Read the model definition and answer for the solid it produces. Units are mm, in the model's axes. A direction names the side the tool comes from. Give positions to 0.01 mm unless a question says otherwise; leave off trailing zeros. Order: outer loops, then holes, each group sorted by start corner. A loop starts at its lowest first (then second) coordinate and runs counter-clockwise, first axis right, second up.
```python
from build123d import *

# Parameters (mm, degrees)
F1_DEPTH = 63.5
F2_DEPTH = 25.4
F3_DEPTH = 8.255
F5_R     = 6.35


with BuildPart() as f1:
    # F0 (on Front) → F1 (new body, symmetric)
    with BuildSketch(Plane.XZ):
        Polygon((41.275, -9.525), (41.275, 9.525), (22.225, 9.525), (-41.275, 9.525), (-41.275, -9.525), align=None)
    extrude(amount=F1_DEPTH, both=True)

    # F0 (on Front) → F2 (join, symmetric)
    with BuildSketch(Plane.XZ):
        with BuildLine():
            Line((22.225, 9.525), (41.275, 9.525))
            Line((41.275, 9.525), (41.275, 27.0002))
            ThreePointArc((41.275, 27.0002), (45.166907, 37.412746), (54.934352, 42.719822))
            Line((54.934352, 42.719822), (54.934352, 61.854849))
            ThreePointArc((54.934352, 61.854849), (31.682991, 50.89972), (22.225, 27.0002))
            Line((22.225, 27.0002), (22.225, 9.525))
        make_face()
        with BuildLine():
            Line((54.934352, 61.854849), (54.934352, 42.719822))
            ThreePointArc((54.934352, 42.719822), (56.039455, 42.836308), (57.15, 42.8752))
            Line((57.15, 42.8752), (85.725, 42.8752))
            Line((85.725, 42.8752), (85.725, 61.9252))
            Line((85.725, 61.9252), (57.15, 61.9252))
            ThreePointArc((57.15, 61.9252), (56.041618, 61.907608), (54.934352, 61.854849))
        make_face()
    extrude(amount=F2_DEPTH, both=True)

    # F0 (on Front) → F3 (join, symmetric)
    with BuildSketch(Plane.XZ):
        with BuildLine():
            Line((-41.275, 9.525), (22.225, 9.525))
            Line((22.225, 9.525), (22.225, 27.0002))
            ThreePointArc((22.225, 27.0002), (31.682991, 50.89972), (54.934352, 61.854849))
            Line((54.934352, 61.854849), (54.934352, 61.970605))
            add(Edge.make_bspline(
                [(-41.275, 9.525), (-22.851193, 36.281686), (-0.588278, 62.756125), (54.934352, 61.970605)],
                knots=[0, 0, 0, 0, 110.052173, 110.052173, 110.052173, 110.052173], degree=3))
        make_face()
    extrude(amount=F3_DEPTH, both=True)

    # F0 (on Front) → F4 (revolve)
    with BuildSketch(Plane.XZ):
        Polygon((85.725, 42.8752), (85.725, 38.1), (105.734352, 38.1), (105.734352, 66.675), (85.725, 66.675), (85.725, 61.9252), align=None)
    revolve(axis=Axis((85.725, 0, 52.3875), (0, 0, 1)))

    # F5
    f5_edges = [f1.edges().sort_by_distance(p)[0] for p in [
        (41.275, -63.5, 0),
        (-41.275, -63.5, 0),
        (-41.275, 63.5, 0),
        (41.275, 63.5, 0),
    ]]
    fillet(f5_edges, radius=F5_R)


solid = f1.part
```
1) The part is cut by section B-B on y = 45. Determine the outline of the cut face in (x, z) (3 decimals), and give its area (3 significant figures).
Final values:
outline: (-41.275, -9.525) - (41.275, -9.525) - (41.275, 9.525) - (-41.275, 9.525) - close
area: 1,570 mm2
2) The part is cut by section A-A on z = 5. Determine the outline of the cut face in (x, y) (3 decimals), and give its area (3 significant figures).
Final values:
outline: (-41.275, -57.15) arc R6.35 ccw to (-34.925, -63.5) - (34.925, -63.5) arc R6.35 ccw to (41.275, -57.15) - (41.275, 57.15) arc R6.35 ccw to (34.925, 63.5) - (-34.925, 63.5) arc R6.35 ccw to (-41.275, 57.15) - close
area: 10,400 mm2
3) Given pin 1 (4.5 mm diameter, centred on y = 23, z = 55, fed in from +X) (3 decimals); pin 2 (6 mm diameter, centred on x = 40, z = -1, fed in from -Y); pin 3 (11 mm diameter, centred on y = -18, z = 2, fed in from +X) (3 decimals), each flat-ended and moving along its own axis, determine where each tip first touches the part or whether it passes through.
Final values:
pin 1: stops at x = 85.725
pin 2: stops at y = -63.15
pin 3: stops at x = 41.275
4) For a pull along X with two mould halves and no side action, classify faces 1 (the face through (1, -36, 9.525)), 2 (the face through (45.06, -0.36, 37.29)), 3 (the face through (65, 0, 42.875)), 4 (the face through (39.464, 61.59, 0.133)) as released by +X, released by -X, zero draft, split by the parting line, or undercut.
Final values:
face 1: zero draft
face 2: undercut
face 3: undercut
face 4: released by +X
5) A tool of negligible diameter and unlimited length cuts with its end or side. For faces 5 (the face through (85.725, -23, 52)), 6 (the face through (46, 25.4, 42)), from which of +Z, -Z, +X, -X, +Y, -Y can it reach the whole face along a straight path? Write none if from no direction.
Final values:
face 5: +Z, -Z, +X, -Y
face 6: +Z, +X, -X, +Y
6) Consider L1, parallel to X at y = -36, z = 4 (3 decimals); L2, parallel to Y at x = 23, z = 55.5 (3 decimals); L3, parallel to Y at x = 37.5, z = 36. Determine where each line is inside the solid, lowest interval first.
Final values:
L1: x = -41.275 to 41.275
L2: y = -8.255 to 8.255
L3: y = -25.4 to 25.4
